from build123d import *

# Parameters (mm, degrees)
SKETCH1_W              = 44.45
SKETCH1_H              = 44.45
BOSS_EXTRUDE1_DEPTH    = 3.175
M2_5_CLEARANCE_HOLE1_D = 2.9
SKETCH5_R              = 7.9375
CUT_EXTRUDE1_DEPTH     = 4.175


with BuildPart() as part:
    # Sketch1 → Boss-Extrude1 (new body)
    with BuildSketch(Plane.XY):
        Rectangle(SKETCH1_W, SKETCH1_H)
    extrude(amount=BOSS_EXTRUDE1_DEPTH)

    # M2.5 Clearance Hole1 (through all)
    with Locations(Plane.XY.offset(3.175)):
        with Locations((-14, 14), (14, -14)):
            Hole(M2_5_CLEARANCE_HOLE1_D / 2)

    # Sketch5 → Cut-Extrude1 (cut, through all)
    with BuildSketch(Plane.XY.offset(3.175)):
        Circle(SKETCH5_R)
    extrude(amount=-CUT_EXTRUDE1_DEPTH, mode=Mode.SUBTRACT)


solid = part.part
Source: CAD feature listing. Evaluate the final solid. Frame: model axes, mm. Round coordinates to 2 decimals unless told otherwise and drop trailing zeros. Loops run counter-clockwise (first coordinate to the right, second up) from the corner with the lowest first, then second, coordinate; pieces in that order, holes last. Notation, with made-up numbers: (-18, 57) -> (-13, 57) arc R33 ccw to (-13, 91) -> close; hole circle Ø1 at (-2.5, 76.5). An arc over 180 degrees is marked (long way). Answer as a JSON object with one key per item and string values. Group by question number.
Q1. Section query C-C (z = 2.1). State how many separate pieces and enclosed holes the cut face has, plus the area to 3 significant figures.
Q2. Section query B-B (x = -14). Output: boundary loops of the cut face in (y, z) (3 decimals), plus the area to 3 significant figures.
Q3. Mould query, pull axis X, two halves, no side actions, for faces 1 (the flat face through (-22.225, 0, 2)), 2 (the flat face through (22.225, 0, 2)), 3 (the cylindrical face through (12.62, -13.56, 1.57)). Classes: pulls with the +X half, pulls with the -X half, needs draft (parallel to the pull), parting line crosses it, or undercut.
Q4. Contact query for a flat-ended pin moving along its axis: P1, Ø2.5, axis at x = 14, y = -14, coming from the -Z side. Output: stop coordinate, or through.
Q5. Section query A-A (y = 14). Output: boundary loops of the cut face in (x, z) (3 decimals).
Q6. Ray query, line 1 (Y direction, x = -14, z = 1.1) (3 decimals); line 2 (Y direction, x = 0, z = 0.7) (1 decimal); line 3 (X direction, y = 2, z = 1.7) (3 decimals). Return the intervals inside material, ascending. Write a range as from..to.
Completed:
{
 "1": {"separate pieces": "1", "enclosed holes": "3", "area": "1,760 mm²"},
 "2": {"outline": "(-22.225, 0) -> (12.55, 0) -> (12.55, 3.175) -> (-22.225, 3.175) -> close; (15.45, 0) -> (22.225, 0) -> (22.225, 3.175) -> (15.45, 3.175) -> close", "area": "132 mm²"},
 "3": {"face 1": "pulls with the -X half", "face 2": "pulls with the +X half", "face 3": "undercut"},
 "4": {"P1": "through"},
 "5": {"outline": "(-22.225, 0) -> (-15.45, 0) -> (-15.45, 3.175) -> (-22.225, 3.175) -> close; (-12.55, 0) -> (22.225, 0) -> (22.225, 3.175) -> (-12.55, 3.175) -> close"},
 "6": {"line 1": "-22.225..12.55, 15.45..22.225", "line 2": "-22.2..-7.9, 7.9..22.2", "line 3": "-22.225..-7.681, 7.681..22.225"}
}
